from build123d import *

# Parameters (mm, degrees)
F0_R     = 50.8
F0_R_2   = 9.525
F1_DEPTH = 44.45
F2_R     = 5.08
F3_R     = 5.08


with BuildPart() as f1:
    # F0 (on Right) → F1 (new body)
    with BuildSketch(Plane.YZ):
        Circle(F0_R)
        Circle(F0_R_2, mode=Mode.SUBTRACT)
    extrude(amount=F1_DEPTH)

    # F2
    f2_edges = [f1.edges().sort_by_distance(p)[0] for p in [
        (44.45, -50.8, 0),
    ]]
    fillet(f2_edges, radius=F2_R)

    # F3
    f3_edges = [f1.edges().sort_by_distance(p)[0] for p in [
        (0, -50.8, 0),
    ]]
    fillet(f3_edges, radius=F3_R)


solid = f1.part
For this review, take the finished solid that the model builds, in its own axes (mm). Give positions to 0.01 mm unless a question says otherwise; leave off trailing zeros. Loops run counter-clockwise (first coordinate to the right, second up) from the corner with the lowest first, then second, coordinate; pieces in that order, holes last. Notation, with made-up numbers: M 77.25,0.25 L 127.25,0.25 A5 ccw 127.25,5.25 Z; hole C 14.5,-30 d9. An arc over 180 degrees is marked long. Answer as a JSON object with one key per item and string values. Group by question number.
Q1. Mouldability with a two-part tool opening along Z and no side actions: class faces 1 (the cylindrical face through (21.914, -7.559, -5.796)), 2 (the cylindrical face through (21.985, -11.012, -49.592)), 3 (the flat face through (44.45, -1, -10)) as +Z half, -Z half, draft (parallel to the pull), parting line (faces both ways), or undercut.
Q2. Add section C-C on x = 22. Give the boundary of the cut face in (y, z) (3 decimals), and give its area (3 significant figures).
Q3. Insertion check: P1, Ø3, axis at x = 38, y = 34.5, coming from the +Z side; P2, Ø1.5, axis at x = 15.5, y = -29.5, coming from the -Z side; P3, Ø6, axis at x = 25.5, z = -8, coming from the -Y side. Each pin has a flat end and moves straight along its axis. Give the tip position at first contact, or say it passes through.
Q4. For probe 1 along Z at (x, y) = (21, 0) (3 decimals); probe 2 along Y at (x, z) = (36, -2.5); probe 3 along Z at (x, y) = (5.5, 29), list the stretches that pass through material, from the lowest coordinate up. Write a range as [from, to].
Q5. Add section D-D on x = 3. Give the boundary of the cut face in (y, z) (3 decimals), and give its area (3 significant figures).
Q6. Add section A-A on z = 0. Give the boundary of the cut face in (x, y) (3 decimals), and give its area (3 significant figures).
Checked values:
{
 "1": {"face 1": "undercut", "face 2": "parting line", "face 3": "draft"},
 "2": {"outline": "C 0,0 d101.6; hole C 0,0 d19.05", "area": "7,820 mm²"},
 "3": {"P1": "z = 38.62", "P2": "z = -41.88", "P3": "y = -50.55"},
 "4": {"probe 1": "[-50.8, -9.525], [9.525, 50.8]", "probe 2": "[-50.74, -9.19], [9.19, 50.74]", "probe 3": "[-41.71, 41.71]"},
 "5": {"outline": "C 0,0 d100.709; hole C 0,0 d19.05", "area": "7,680 mm²"},
 "6": {"outline": "M 0,-45.72 A5.08 ccw 5.08,-50.8 L 39.37,-50.8 A5.08 ccw 44.45,-45.72 L 44.45,-9.525 L 0,-9.525 Z; M 0,9.525 L 44.45,9.525 L 44.45,45.72 A5.08 ccw 39.37,50.8 L 5.08,50.8 A5.08 ccw 0,45.72 Z", "area": "3,650 mm²"}
}
